For this review, take the finished solid that the model builds, in its own axes (mm). A direction names the side the tool comes from. Coordinates: 2 decimals unless noted, no trailing zeros. Write each loop counter-clockwise with the first axis right and the second up, starting at its lowest first coordinate (ties: lowest second). Pieces come first, ordered by that corner, then holes. Notation, with made-up numbers: (45.5, 43) - (79.5, 43) arc R25 ccw to (79.5, 66) - close; hole circle Ø4 at (87, -40). An arc over 180 degrees is marked (long way). Use one line per item in the form item = value. Start each with the question number.
1) Insertion check: P1, Ø1, axis at x = -2, z = 11.5, coming from the -Y side; P2, Ø2, axis at y = 6, z = 1.5, coming from the -X side; P3, Ø2.5, axis at x = 12, y = 7, coming from the +Z side; P4, Ø2, axis at x = 9, y = 8, coming from the +Z side. Each pin has a flat end and moves straight along its axis. Give the tip position at first contact, or say it passes through.
2) For L1, parallel to Z at x = -2.25, y = 9.25; L2, parallel to X at y = 5.75, z = 0; L3, parallel to X at y = 3.5, z = -7, list the stretches that pass through material, from the lowest coordinate up. Write a range as from..to.
3) Tool access review of faces 4 (the flat face through (-3.219, 5.151, 5.474)), 5 (the flat face through (10, 5, -1.016)), 6 (the flat face through (-3, 10.16, 6)): name each direction out of +Z, -Z, +X, -X, +Y, -Y from which nothing blocks a thin tool from reaching the whole face with its end or side.
4) We need section D-D (z = 0). Give the boundary of the cut face in (x, y), plus the area to 3 significant figures.
5) Mouldability with a two-part tool opening along X and no side actions: class faces 1 (the flat face through (6.35, 5, -2)), 2 (the flat face through (-11.112, 5, 0)), 3 (the flat face through (-9, 5, 1.016)) as pulls with the +X half, pulls with the -X half, needs draft (parallel to the pull), parting line crosses it, or undercut.
6) We need section B-B (x = 8.25). Give the boundary of the cut face in (y, z).
7) We need section A-A (z = 3). Give the boundary of the cut face in (x, y).
```python
from build123d import *

# Parameters (mm, degrees)
SKETCH1_R           = 14.2875
BOSS_EXTRUDE1_DEPTH = 10.16
CUT_EXTRUDE1_DEPTH  = 23.61616485
SKETCH3_W           = 25.4
SKETCH3_H           = 2.032
CUT_EXTRUDE2_DEPTH  = 23.61616485


with BuildPart() as part:
    # Sketch1 → Boss-Extrude1 (new body)
    with BuildSketch(Plane(origin=(0, 0, 0), x_dir=(1, 0, 0), z_dir=(0, 1, 0))):
        with Locations(Location((0, 0, 0), (0, 0, 270))):
            Circle(SKETCH1_R)
    extrude(amount=BOSS_EXTRUDE1_DEPTH)

    # Sketch2 → Cut-Extrude1 (cut, through all)
    with BuildSketch(Plane(origin=(0, 10.16, 0), x_dir=(1, 0, 0), z_dir=(0, 1, 0))):
        Polygon((0, 7.332348419), (-6.35, 3.666174209), (-6.35, -3.666174209), (0, -7.332348419), (6.35, -3.666174209), (6.35, 3.666174209), align=None)
    extrude(amount=-CUT_EXTRUDE1_DEPTH, mode=Mode.SUBTRACT)

    # Sketch3 → Cut-Extrude2 (cut, through all)
    with BuildSketch(Plane(origin=(0, 10.16, 0), x_dir=(1, 0, 0), z_dir=(0, 1, 0))):
        with Locations((1.5875, 0)):
            Rectangle(SKETCH3_W, SKETCH3_H)
    extrude(amount=-CUT_EXTRUDE2_DEPTH, mode=Mode.SUBTRACT)


solid = part.part
```
Determined:
q1.P1 = 0
q1.P2 = -14.28
q1.P3 = 9.41
q1.P4 = 11.84
q2.L1 = -14.11..-6.03, 6.03..14.11
q2.L2 = -14.29..-11.11
q2.L3 = -12.46..-0.58, 0.58..12.46
q3.face_4 = +Y, -Y
q3.face_5 = +X, +Y, -Y
q3.face_6 = +Z, -Z, +X, -X, +Y
q4.outline = (-14.29, 0) - (-11.11, 0) - (-11.11, 10.16) - (-14.29, 10.16) - close
q4.area = 32.3 mm²
q5.face_1 = undercut
q5.face_2 = pulls with the +X half
q5.face_3 = needs draft
q6.outline = (0, -11.66) - (10.16, -11.66) - (10.16, -1.02) - (0, -1.02) - close; (0, 1.02) - (10.16, 1.02) - (10.16, 11.66) - (0, 11.66) - close
q7.outline = (-13.97, 0) - (-6.35, 0) - (-6.35, 10.16) - (-13.97, 10.16) - close; (6.35, 0) - (13.97, 0) - (13.97, 10.16) - (6.35, 10.16) - close
